Input: part model. Units: mm. Frame: model coordinates. A direction names the side the tool comes from. Round coordinates to 2 decimals unless told otherwise and drop trailing zeros. Loops run counter-clockwise (first coordinate to the right, second up) from the corner with the lowest first, then second, coordinate; pieces in that order, holes last. Notation, with made-up numbers: (-16, 71.5) -> (35, 71.5) arc R18 cw to (35, 90.5) -> close; hole circle Ø2 at (87.25, -15.5). An arc over 180 degrees is marked (long way). Answer as a JSON object with one key per item and string values. Group by question number.
Item 1: Draft query along Z for faces 3 (the flat face through (-3, 3.9, -2)), 4 (the cylindrical face through (6.466, 0.222, 2.681)), 5 (the cylindrical face through (-2.579, 1.977, 1.978)). Return one class per face: released by +Z, released by -Z, zero draft, split by the parting line, or undercut.
Item 2: Section query C-C on y = 1.1. Return loops of the section in (x, z), and give its area (3 significant figures).
Item 3: Set-up query: faces 1 (the cylindrical face through (6.466, 3.672, 2.681)), 2 (the flat face through (3, 3.45, -5)). Return all of +Z, -Z, +X, -X, +Y, -Y with unobstructed straight access to the full face (end or side cutting, diameter ignored); none if empty.
Item 4: Material intervals for line 1 (X direction, y = 1.7, z = 0); line 2 (Y direction, x = -5.5, z = -4), sorted ascending. Write a range as [from, to].
Item 5: Section query B-B on x = 0. Return loops of the section in (y, z).
Item 6: Section query A-A on z = 0. Return loops of the section in (x, y), and give its area (3 significant figures).
Item 7: Pin query (flat end, axial travel): pin 1 (2 mm diameter, centred on x = 4, y = 3, fed in from -Z); pin 2 (1 mm diameter, centred on y = 2, z = -3, fed in from +X). Return the tip coordinate at first contact, or that it passes through.
from build123d import *


with BuildPart() as part:
    # ｽｹｯﾁ1 → 回転1 (revolve)
    with BuildSketch(Plane.XY):
        with BuildLine():
            Line((7, 3.45), (5.3, 3.45))
            ThreePointArc((5.3, 3.45), (5.087867966, 3.362132034), (5, 3.15))
            Line((5, 3.15), (5, 0.75))
            ThreePointArc((5, 0.75), (5.087867966, 0.537867966), (5.3, 0.45))
            Line((5.3, 0.45), (7, 0.45))
            Line((7, 0.45), (7, 0))
            Line((7, 0), (3.25, 0))
            Line((3.25, 0), (3.25, 3.9))
            Line((3.25, 3.9), (7, 3.9))
            Line((7, 3.9), (7, 3.45))
        make_face()
    revolve(axis=Axis((0, 1.95, 0), (0, 1, 0)))


solid = part.part
Solved:
{
 "1": {"face 3": "zero draft", "face 4": "split by the parting line", "face 5": "undercut"},
 "2": {"outline": "circle Ø10 at (0, 0); hole circle Ø6.5 at (0, 0)", "area": "45.4 mm²"},
 "3": {"face 1": "+Y, -Y", "face 2": "none"},
 "4": {"line 1": "[-5, -3.25], [3.25, 5]", "line 2": "[0, 0.45], [3.45, 3.9]"},
 "5": {"outline": "(0, -7) -> (0.45, -7) -> (0.45, -5.3) arc R0.3 cw to (0.75, -5) -> (3.15, -5) arc R0.3 cw to (3.45, -5.3) -> (3.45, -7) -> (3.9, -7) -> (3.9, -3.25) -> (0, -3.25) -> close; (0, 3.25) -> (3.9, 3.25) -> (3.9, 7) -> (3.45, 7) -> (3.45, 5.3) arc R0.3 cw to (3.15, 5) -> (0.75, 5) arc R0.3 cw to (0.45, 5.3) -> (0.45, 7) -> (0, 7) -> close"},
 "6": {"outline": "(-7, 0) -> (-3.25, 0) -> (-3.25, 3.9) -> (-7, 3.9) -> (-7, 3.45) -> (-5.3, 3.45) arc R0.3 cw to (-5, 3.15) -> (-5, 0.75) arc R0.3 cw to (-5.3, 0.45) -> (-7, 0.45) -> close; (3.25, 0) -> (7, 0) -> (7, 0.45) -> (5.3, 0.45) arc R0.3 cw to (5, 0.75) -> (5, 3.15) arc R0.3 cw to (5.3, 3.45) -> (7, 3.45) -> (7, 3.9) -> (3.25, 3.9) -> close", "area": "17.3 mm²"},
 "7": {"pin 1": "z = -6.27", "pin 2": "x = 4.33"}
}
